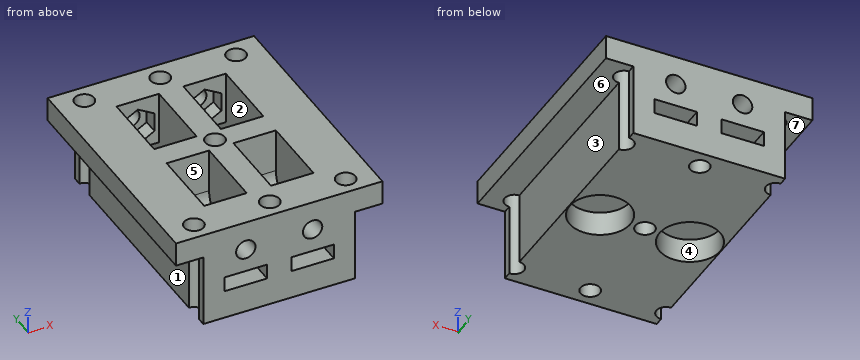
```python
from build123d import *

# Parameters (mm, degrees)
PAD_DEPTH         = 20.5
SKETCH001_R       = 1.6
POCKET_DEPTH      = 16.001
POCKET_DEPTH_BACK = 0.001
POCKET001_DEPTH   = 7
POCKET002_DEPTH   = 1
POCKET003_DEPTH   = 7
SKETCH005_R       = 1.6
POCKET004_DEPTH   = 6.501
POCKET005_DEPTH   = 2.5
SKETCH007_R       = 1.6
POCKET006_DEPTH   = 6.501
POCKET007_DEPTH   = 2.5
SKETCH009_R       = 5
POCKET008_DEPTH   = 4


with BuildPart() as part:
    # Sketch → Pad (new body, symmetric)
    with BuildSketch(Plane.XZ):
        Polygon((12.5, 6), (12.5, -6), (-12.5, -6), (-12.5, 6), (-17, 6), (-17, 10), (17, 10), (17, 6), align=None)
    extrude(amount=PAD_DEPTH, both=True)

    # Sketch001 (on Face6 of Pad) → Pocket (cut, two sides)
    with BuildSketch(Plane(origin=(0, 0, 10), x_dir=(-1, 0, 0), z_dir=(0, 0, 1))) as pocket_sk:
        with Locations((-12.5, 17.5)):
            Circle(SKETCH001_R)
        with Locations((12.5, 17.5)):
            Circle(SKETCH001_R)
        with Locations((0, 17.5)):
            Circle(SKETCH001_R)
        with Locations((-12.5, -17.5)):
            Circle(SKETCH001_R)
        with Locations((12.5, -17.5)):
            Circle(SKETCH001_R)
        Circle(SKETCH001_R)
        with Locations((0, -17.5)):
            Circle(SKETCH001_R)
    extrude(amount=-POCKET_DEPTH, mode=Mode.SUBTRACT)
    extrude(pocket_sk.sketch, amount=POCKET_DEPTH_BACK, mode=Mode.SUBTRACT)

    # Sketch002 (on DatumPlane) → Pocket001 (cut)
    with BuildSketch(Plane.YZ.offset(2)):
        with BuildLine():
            ThreePointArc((-6, -1.25), (-3.171573, -0.078427), (-2, 2.75))
            Line((-2, 2.75), (-2, 10))
            Line((-14, 10), (-2, 10))
            Line((-14, 10), (-14, 1.25))
            Line((-14, 1.25), (-20.5, 1.25))
            Line((-20.5, 1.25), (-20.5, -1.25))
            Line((-20.5, -1.25), (-6, -1.25))
        make_face()
        with BuildLine():
            ThreePointArc((2, 2.75), (3.171573, -0.078427), (6, -1.25))
            Line((20.5, -1.25), (6, -1.25))
            Line((20.5, 1.25), (20.5, -1.25))
            Line((14, 1.25), (20.5, 1.25))
            Line((14, 10), (14, 1.25))
            Line((2, 10), (14, 10))
            Line((2, 2.75), (2, 10))
        make_face()
    extrude(amount=POCKET001_DEPTH, mode=Mode.SUBTRACT)

    # Sketch001 (on Face6 of Pad) → Pocket002 (cut)
    with BuildSketch(Plane(origin=(0, 0, 10), x_dir=(-1, 0, 0), z_dir=(0, 0, 1))):
        with Locations((-12.5, 17.5)):
            Circle(SKETCH001_R)
        with Locations((12.5, 17.5)):
            Circle(SKETCH001_R)
        with Locations((0, 17.5)):
            Circle(SKETCH001_R)
        with Locations((-12.5, -17.5)):
            Circle(SKETCH001_R)
        with Locations((12.5, -17.5)):
            Circle(SKETCH001_R)
        Circle(SKETCH001_R)
        with Locations((0, -17.5)):
            Circle(SKETCH001_R)
    extrude(amount=-POCKET002_DEPTH, mode=Mode.SUBTRACT)

    # Sketch004 (on DatumPlane) → Pocket003 (cut)
    with BuildSketch(Plane.YZ.offset(-2)):
        with BuildLine():
            ThreePointArc((-6, -1.25), (-3.171573, -0.078427), (-2, 2.75))
            Line((-2, 10), (-2, 2.75))
            Line((-2, 10), (-14, 10))
            Line((-14, 10), (-14, 1.25))
            Line((-14, 1.25), (-20.5, 1.25))
            Line((-20.5, 1.25), (-20.5, -1.25))
            Line((-20.5, -1.25), (-6, -1.25))
        make_face()
        with BuildLine():
            ThreePointArc((2, 2.75), (3.171573, -0.078427), (6, -1.25))
            Line((20.5, -1.25), (6, -1.25))
            Line((20.5, 1.25), (20.5, -1.25))
            Line((14, 1.25), (20.5, 1.25))
            Line((14, 10), (14, 1.25))
            Line((2, 10), (14, 10))
            Line((2, 2.75), (2, 10))
        make_face()
    extrude(amount=-POCKET003_DEPTH, mode=Mode.SUBTRACT)

    # Sketch005 (on DatumPlane) → Pocket004 (cut, through all)
    with BuildSketch(Plane.XZ.offset(14)):
        with Locations((-5.5, 5.125)):
            Circle(SKETCH005_R)
        with Locations((5.5, 5.125)):
            Circle(SKETCH005_R)
    extrude(amount=POCKET004_DEPTH, mode=Mode.SUBTRACT)

    # Sketch006 (on DatumPlane) → Pocket005 (cut)
    with BuildSketch(Plane.XZ.offset(14)):
        Polygon((-2.750142, 3.537404), (-2.750142, 6.71283), (-5.500142, 8.300543), (-8.250142, 6.71283), (-8.250142, 3.537404), (-5.500142, 1.94969), align=None)
        Polygon((9.85, 3.537287), (9.85, 6.712713), (7.1, 8.300426), (4.35, 6.712713), (4.35, 3.537287), (7.1, 1.949574), align=None)
    extrude(amount=POCKET005_DEPTH, mode=Mode.SUBTRACT)

    # Sketch007 (on DatumPlane) → Pocket006 (cut, through all)
    with BuildSketch(Plane.XZ.offset(-14)):
        with Locations((-5.5, 5.125)):
            Circle(SKETCH007_R)
        with Locations((5.5, 5.125)):
            Circle(SKETCH007_R)
    extrude(amount=-POCKET006_DEPTH, mode=Mode.SUBTRACT)

    # Sketch008 (on DatumPlane) → Pocket007 (cut)
    with BuildSketch(Plane.XZ.offset(-14)):
        Polygon((-2.75, 3.537287), (-2.75, 6.712713), (-5.5, 8.300426), (-8.25, 6.712713), (-8.25, 3.537287), (-5.5, 1.949574), align=None)
        Polygon((8.25, 3.537287), (8.25, 6.712713), (5.5, 8.300426), (2.75, 6.712713), (2.75, 3.537287), (5.5, 1.949574), align=None)
    extrude(amount=-POCKET007_DEPTH, mode=Mode.SUBTRACT)

    # Sketch009 (on DatumPlane) → Pocket008 (cut)
    with BuildSketch(Plane.XY.offset(-6)):
        with Locations((-7.4, 0)):
            Circle(SKETCH009_R)
        with Locations((7.4, 0)):
            Circle(SKETCH009_R)
    extrude(amount=POCKET008_DEPTH, mode=Mode.SUBTRACT)


solid = part.part
```
For this review, take the finished solid that the model builds, in its own axes (mm). Face numbers are marked on the shaded views. A direction names the side the tool comes from. Round coordinates to 2 decimals unless told otherwise and drop trailing zeros. Loops run counter-clockwise (first coordinate to the right, second up) from the corner with the lowest first, then second, coordinate; pieces in that order, holes last.
Q1. Add section C-C on z = 0. Give the number of separate pieces and of enclosed holes in the cut face, plus the area to 3 significant figures.
Result sheet:
separate pieces: 1
enclosed holes: 3
area: 497 mm2
Q2. To check wall thickness, follow line 1 along Y through (x, z) = (0, 4.75); line 2 along Y through (x, z) = (-5.5, 9.25); line 3 along Y through (x, z) = (8, 3.75). State the ranges of each line that lie inside material, in increasing order.
Result sheet:
line 1: y = -20.5 to -19.1, -15.9 to -1.6, 1.6 to 15.9, 19.1 to 20.5
line 2: y = -20.5 to -14, -2 to 2, 14 to 20.5
line 3: y = -20.5 to -16.5, -2 to 2, 16.5 to 20.5
Q3. Add section B-B on y = 18. Write out the cut boundary in (x, z) (3 decimals).
Result sheet:
outline: (-17, 6) - (-14.02, 6) - (-14.02, 10) - (-17, 10) - close; (-10.98, -6) - (-1.52, -6) - (-1.52, 10) - (-10.98, 10) - close; (1.52, -6) - (10.98, -6) - (10.98, 10) - (1.52, 10) - close; (14.02, 6) - (17, 6) - (17, 10) - (14.02, 10) - close; hole (-9, -1.25) - (-2, -1.25) - (-2, 1.25) - (-9, 1.25) - close; hole circle Ø3.2 at (-5.5, 5.125); hole (2, -1.25) - (9, -1.25) - (9, 1.25) - (2, 1.25) - close; hole circle Ø3.2 at (5.5, 5.125)
Q4. Insertion check: pin 1 Ø2 at (y, z) = (-3.5, -2.5) entering from -X; pin 2 Ø1.1 at (y, z) = (-19.5, -1.5) entering from +X; pin 3 Ø5 at (x, y) = (7.5, 1) entering from -Z. Each pin has a flat end and moves straight along its axis. Give the tip position at first contact, or say it passes through.
Result sheet:
pin 1: stops at x = -12.5
pin 2: stops at x = 12.5
pin 3: stops at z = -2
Q5. Add section A-A on y = 0. Write out the cut boundary in (x, z).
Result sheet:
outline: (-17, 6) - (-12.5, 6) - (-12.5, -6) - (-12.4, -6) - (-12.4, -2) - (-2.4, -2) - (-2.4, -6) - (-1.6, -6) - (-1.6, 10) - (-17, 10) - close; (1.6, -6) - (2.4, -6) - (2.4, -2) - (12.4, -2) - (12.4, -6) - (12.5, -6) - (12.5, 6) - (17, 6) - (17, 10) - (1.6, 10) - close
Q6. Mouldability with a two-part tool opening along X and no side actions: class the marked faces 1, 2 and 3 as +X half, -X half, draft (parallel to the pull), parting line (faces both ways), or undercut.
Result sheet:
face 1: -X half
face 2: undercut
face 3: +X half
Q7. Add section D-D on x = -15. Write out the cut boundary in (y, z), plus the area to 3 significant figures.
Result sheet:
outline: (-20.5, 6) - (20.5, 6) - (20.5, 10) - (-20.5, 10) - close
area: 164 mm2
Q8. Machinability: for the marked faces 4, 5, 6 and 7, which of the approach directions +Z, -Z, +X, -X, +Y, -Y give a long, thin tool a straight path to every point of the face, cutting with its end or side? Answer none if there is none.
Result sheet:
face 4: -Z
face 5: +Z
face 6: -Z, +X, +Y, -Y
face 7: -Z, -X, +Y, -Y
